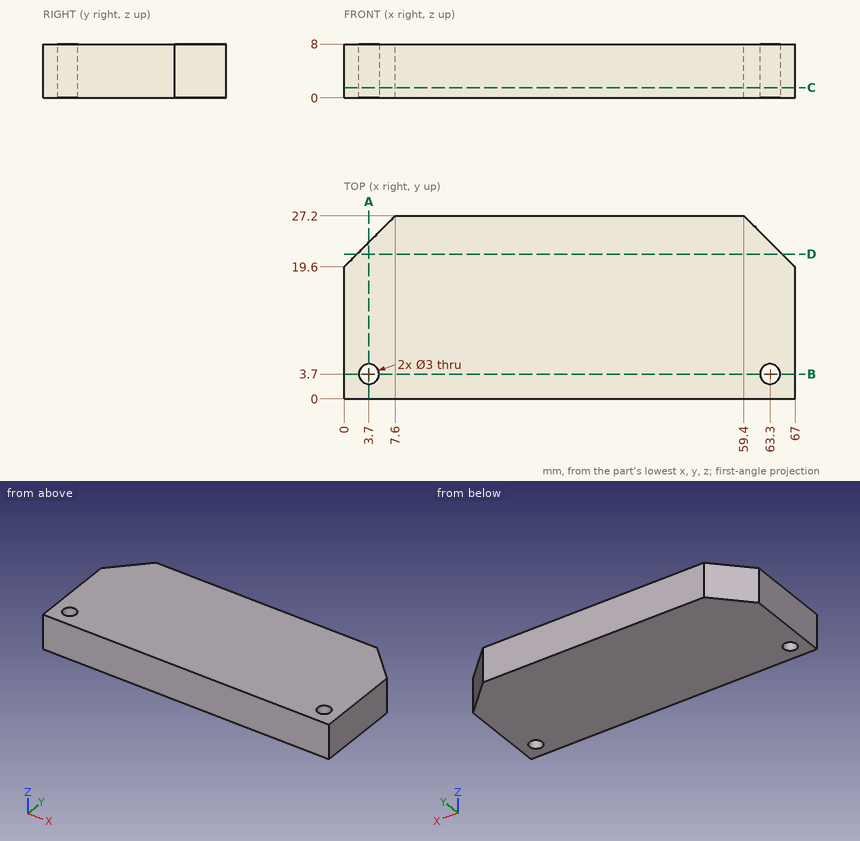
Check sheet for the drawn part. Datum: minimum x, y, z corner. Units: mm. Round coordinates to 2 decimals unless told otherwise and drop trailing zeros. Loops run counter-clockwise (first coordinate to the right, second up) from the corner with the lowest first, then second, coordinate; pieces in that order, holes last. Notation, with made-up numbers: (24, -11.5) - (72, -11.5) arc R13 cw to (72, 8.5) - close; hole circle Ø9 at (17, 49.25). An arc over 180 degrees is marked (long way). Write item = value, one per line. Start each with the question number.
1. Section check D-D on y = 21.5. Enter the section's corners in (x, z), then the cut area to 3 significant figures.
2. Section check C-C on z = 1.5. Enter the section's corners in (x, y), then the cut area to 3 significant figures.
3. Section check B-B on y = 3.7. Enter the section's corners in (x, z), then the cut area to 3 significant figures.
4. Section check A-A on x = 3.7. Enter the section's corners in (y, z), then the cut area to 3 significant figures.
5. Thickness scan on line 1 (Y direction, x = 3.7, z = 2); line 2 (Y direction, x = 64, z = 2.75); line 3 (X direction, y = 22.25, z = 7). Record the ranges inside material, lowest first.
Working result:
q1.outline = (1.9, 0) - (65.1, 0) - (65.1, 8) - (1.9, 8) - close
q1.area = 506 mm^2
q2.outline = (0, 0) - (67, 0) - (67, 19.6) - (59.4, 27.2) - (7.6, 27.2) - (0, 19.6) - close; hole circle Ø3 at (3.7, 3.7); hole circle Ø3 at (63.3, 3.7)
q2.area = 1,750 mm^2
q3.outline = (0, 0) - (2.2, 0) - (2.2, 8) - (0, 8) - close; (5.2, 0) - (61.8, 0) - (61.8, 8) - (5.2, 8) - close; (64.8, 0) - (67, 0) - (67, 8) - (64.8, 8) - close
q3.area = 488 mm^2
q4.outline = (0, 0) - (2.2, 0) - (2.2, 8) - (0, 8) - close; (5.2, 0) - (23.3, 0) - (23.3, 8) - (5.2, 8) - close
q4.area = 162 mm^2
q5.line_1 = 0 to 2.2, 5.2 to 23.3
q5.line_2 = 0 to 2.37, 5.03 to 22.6
q5.line_3 = 2.65 to 64.35
